Design review of the part shown in the three views and the two pictorial views. Dimensions are in mm from the part's minimum x, y and z. A direction names the side the tool comes from. Round coordinates to 2 decimals unless told otherwise and drop trailing zeros. Loops run counter-clockwise (first coordinate to the right, second up) from the corner with the lowest first, then second, coordinate; pieces in that order, holes last. Notation, with made-up numbers: (41, -22.5) -> (77, -22.5) arc R11 cw to (77, -18.5) -> close; hole circle Ø11 at (23, -16). An arc over 180 degrees is marked (long way). One line per question, with ' | ' between items. Start each with the question number.
1. For the marked faces 1 and 2, list the 3-axis set-ups (+Z, -Z, +X, -X, +Y, -Y) from which the entire face can be reached by the end or side of a thin tool; tool diameter is ignored.
2. For pin 1 Ø1.5 at (y, z) = (25.5, 9.5) entering from -X; pin 2 Ø4 at (y, z) = (12.5, 49) entering from +X; pin 3 Ø19 at (x, y) = (47, 11) entering from +Z, all flat-tipped, find the tip position at first contact; note any pin that passes through.
3. Wall thickness on line 1 along X through (y, z) = (19, 2) (3 decimals); line 2 along X through (y, z) = (12.5, 4) (3 decimals); line 3 along Z through (x, y) = (5, 23) (3 decimals): over which ranges is each line inside the solid? List them lowest first.
4. Consider section C-C (z = 53). Write out the cut boundary in (x, y) (3 decimals), and give its area (3 significant figures).
5. Consider section D-D (x = 33). Write out the cut boundary in (y, z) (3 decimals), and give its area (3 significant figures).
6. Consider section B-B (y = 19.05). Write out the cut boundary in (x, z) (3 decimals), and give its area (3 significant figures).
7. Consider section A-A (y = 26.5). Write out the cut boundary in (x, z) (3 decimals).
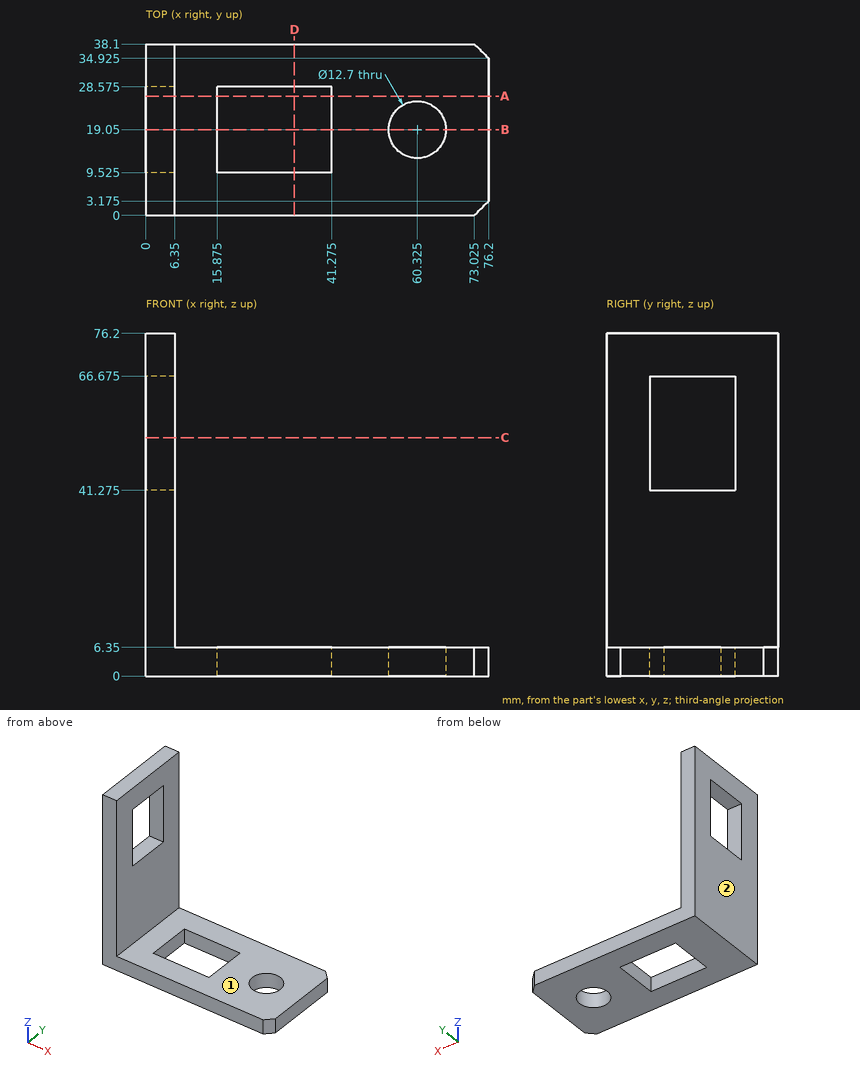
Answer block:
1) face 1: +Z, +X, +Y, -Y | face 2: +Z, -Z, -X, +Y, -Y
2) pin 1: stops at x = 0 | pin 2: passes through | pin 3: stops at z = 6.35
3) line 1: x = 0 to 15.875, 41.275 to 53.975, 66.675 to 76.2 | line 2: x = 0 to 15.875, 41.275 to 76.2 | line 3: z = 0 to 41.275, 66.675 to 76.2
4) outline: (0, 0) -> (6.35, 0) -> (6.35, 9.525) -> (0, 9.525) -> close; (0, 28.575) -> (6.35, 28.575) -> (6.35, 38.1) -> (0, 38.1) -> close | area: 121 mm2
5) outline: (0, 0) -> (9.525, 0) -> (9.525, 6.35) -> (0, 6.35) -> close; (28.575, 0) -> (38.1, 0) -> (38.1, 6.35) -> (28.575, 6.35) -> close | area: 121 mm2
6) outline: (0, 0) -> (15.875, 0) -> (15.875, 6.35) -> (6.35, 6.35) -> (6.35, 41.275) -> (0, 41.275) -> close; (0, 66.675) -> (6.35, 66.675) -> (6.35, 76.2) -> (0, 76.2) -> close; (41.275, 0) -> (53.975, 0) -> (53.975, 6.35) -> (41.275, 6.35) -> close; (66.675, 0) -> (76.2, 0) -> (76.2, 6.35) -> (66.675, 6.35) -> close | area: 524 mm2
7) outline: (0, 0) -> (15.875, 0) -> (15.875, 6.35) -> (6.35, 6.35) -> (6.35, 41.275) -> (0, 41.275) -> close; (0, 66.675) -> (6.35, 66.675) -> (6.35, 76.2) -> (0, 76.2) -> close; (41.275, 0) -> (76.2, 0) -> (76.2, 6.35) -> (41.275, 6.35) -> close
